```python
from build123d import *

# Parameters (mm, degrees)
F0_R     = 13.5
F1_DEPTH = 1
F2_R     = 12.5
F3_DEPTH = 5
F4_R     = 6.1
F5_DEPTH = 6.001


with BuildPart() as f1:
    # F0 (on Top) → F1 (new body)
    with BuildSketch(Plane.XY):
        Circle(F0_R)
    extrude(amount=F1_DEPTH)

    # F2 (on face) → F3 (join)
    with BuildSketch(Plane(origin=(0, 0, 0), x_dir=(1, 0, 0), z_dir=(0, 0, -1))):
        Circle(F2_R)
    extrude(amount=F3_DEPTH)

    # F4 (on face) → F5 (cut, through all)
    with BuildSketch(Plane.XY.offset(1)):
        Circle(F4_R)
    extrude(amount=-F5_DEPTH, mode=Mode.SUBTRACT)


solid = f1.part
```
Design review of the part built by this model. Coordinates are the model's own, in mm. A direction names the side the tool comes from. Give positions to 0.01 mm unless a question says otherwise; leave off trailing zeros. Write each loop counter-clockwise with the first axis right and the second up, starting at its lowest first coordinate (ties: lowest second). Pieces come first, ordered by that corner, then holes. Notation, with made-up numbers: (28, 84) -> (45, 84) arc R18 cw to (45, 94) -> close; hole circle Ø11 at (-8, 74). An arc over 180 degrees is marked (long way). Answer in a Markdown table with one row per item.
(1) Consider section D-D (x = -11.5). State the section outline as (y, z) points, then the cut area to 3 significant figures.
Results:
| item | result |
|---|---|
| outline | (-7.07, 0) -> (-4.9, 0) -> (-4.9, -5) -> (4.9, -5) -> (4.9, 0) -> (7.07, 0) -> (7.07, 1) -> (-7.07, 1) -> close |
| area | 63.1 mm2 |
(2) Consider section C-C (z = -2.4). State the section outline as (x, y) points.
Results:
| item | result |
|---|---|
| outline | circle Ø25 at (0, 0); hole circle Ø12.2 at (0, 0) |
(3) Consider section A-A (y = 0). State the section outline as (x, z) points, then the cut area to 3 significant figures.
Results:
| item | result |
|---|---|
| outline | (-13.5, 0) -> (-12.5, 0) -> (-12.5, -5) -> (-6.1, -5) -> (-6.1, 1) -> (-13.5, 1) -> close; (6.1, -5) -> (12.5, -5) -> (12.5, 0) -> (13.5, 0) -> (13.5, 1) -> (6.1, 1) -> close |
| area | 78.8 mm2 |
(4) For faces 1 (the cylindrical face through (11.923, -3.755, -2.465)), 2 (the flat face through (6, -3, 1)), list the 3-axis set-ups (+Z, -Z, +X, -X, +Y, -Y) from which the entire face can be reached by the end or side of a thin tool; tool diameter is ignored.
Results:
| item | result |
|---|---|
| face 1 | -Z |
| face 2 | +Z, +X, -X, +Y, -Y |
(5) To check wall thickness, follow probe 1 along Y at (x, z) = (0, -1.65); probe 2 along Z at (x, y) = (-9.5, 9); probe 3 along Y at (x, z) = (4.5, 0.05). State the ranges of each line that lie inside material, in increasing order.
Results:
| item | result |
|---|---|
| probe 1 | -12.5 to -6.1, 6.1 to 12.5 |
| probe 2 | 0 to 1 |
| probe 3 | -12.73 to -4.12, 4.12 to 12.73 |
(6) Mouldability with a two-part tool opening along Y and no side actions: class faces 3 (the cylindrical face through (-2.93, -13.18, 0.49)), 4 (the flat face through (9, -9, 0)), 5 (the cylindrical face through (-6.094, 0.268, -1.958)) as +Y half, -Y half, draft (parallel to the pull), parting line (faces both ways), or undercut.
Results:
| item | result |
|---|---|
| face 3 | parting line |
| face 4 | draft |
| face 5 | undercut |
(7) Clearance check with flat-ended pins moving along their axes: pin 1 (1.5 mm diameter, centred on x = -8, z = -2.5, fed in from +Y); pin 2 (1.5 mm diameter, centred on x = -2.5, z = -3, fed in from -Y); pin 3 (1 mm diameter, centred on y = 7.5, z = 0.5, fed in from +X). State where each tip first meets the part, or that it passes through.
Results:
| item | result |
|---|---|
| pin 1 | y = 10.18 |
| pin 2 | y = -12.38 |
| pin 3 | x = 11.54 |
